Model file for the job. Use its own axes, mm. A direction names the side the tool comes from. Coordinates: 2 decimals unless noted, no trailing zeros. Write each loop counter-clockwise with the first axis right and the second up, starting at its lowest first coordinate (ties: lowest second). Pieces come first, ordered by that corner, then holes.
Q1. Band-saw the part on B-B, the plane x = -2. Write the cut outline in (y, z).
Q2. Band-saw the part on D-D, the plane x = 9.5. Write the cut outline in (y, z).
Q3. Pin check, flat tips, straight feed: P1, Ø6, axis at y = 16, z = -14, coming from the +X side; P2, Ø1.5, axis at x = 13.5, z = 7, coming from the +Y side; P3, Ø4, axis at y = 13.5, z = -22.5, coming from the -X side. Stop position of each tip, or through.
Q4. Band-saw the part on C-C, the plane z = -21. Write the cut outline in (x, y), plus the area to 3 significant figures.
Q5. Pull direction X, two halves, no side cores. Call faces 1 (the cylindrical face through (-29.4, 15.18, 29.43)), 2 (the flat face through (0, 1.5, 0)), 3 (the cylindrical face through (29.43, 15.18, 29.4)), 4 (the flat face through (-31, 2, -1)): released by +X, released by -X, zero draft, split by the parting line, or undercut.
Q6. Drill centre lines: probe 1 along Z at (x, y) = (-19.5, 11); probe 2 along Y at (x, z) = (23, 11). Where is each one in solid material? Low to high.
Q7. Which spindle directions (+Z, -Z, +X, -X, +Y, -Y) get a long thin tool onto all of the face, cutting with end or side? Do faces 5 (the flat face through (0, 15, 30)), 6 (the flat face through (0, 15, -28.5)), 7 (the flat face through (31, 2, -1)). Say none if no direction does.
from build123d import *

# Parameters (mm, degrees)
SKETCH_1_W            = 60
SKETCH_1_H            = 60
EXTRUDE_1_DEPTH       = 28
SKETCH_2_W            = 57
SKETCH_2_H            = 57
CUT_EXTRUDE_1_DEPTH   = 26.5
EXTRUDE_3_DEPTH       = 26
MIRROR_5_COPY_1_DEPTH = 26
SKETCH_4_W            = 8
SKETCH_4_H            = 2
CUT_EXTRUDE_2_DEPTH   = 2
FILLET_1_R            = 2


with BuildPart() as part:
    # 草图1 → 凸台-拉伸1 (new body)
    with BuildSketch(Plane(origin=(0, 0, 0), x_dir=(1, 0, 0), z_dir=(0, 1, 0))):
        Rectangle(SKETCH_1_W, SKETCH_1_H)
    extrude(amount=EXTRUDE_1_DEPTH)

    # 草图2 → 切除-拉伸1 (cut)
    with BuildSketch(Plane(origin=(0, 28, 0), x_dir=(1, 0, 0), z_dir=(0, 1, 0))):
        Rectangle(SKETCH_2_W, SKETCH_2_H)
    extrude(amount=-CUT_EXTRUDE_1_DEPTH, mode=Mode.SUBTRACT)

    # 草图3 → 凸台-拉伸3 (add)
    with BuildSketch(Plane(origin=(0, 28, 0), x_dir=(1, 0, 0), z_dir=(0, 1, 0))):
        with BuildLine():
            Line((-30, 0), (-30, -1.5))
            Line((-30, -1.5), (-30.677124344, -1.5))
            ThreePointArc((-30.677124344, -1.5), (-31.088161527, -1.780042303), (-31.555590279, -1.95))
            Line((-31.555590279, -1.95), (-32.5, -1.95))
            Line((-32.5, -1.95), (-32.5, -1.443375673))
            Line((-32.5, -1.443375673), (-30, 0))
        make_face()
    extrude_3 = extrude(amount=-EXTRUDE_3_DEPTH)

    # 镜向4: 凸台-拉伸3 across plane
    add(extrude_3.mirror(Plane.XY))

    # 镜向5: 凸台-拉伸3 across plane
    add(extrude_3.mirror(Plane(origin=(0, 0, 0), x_dir=(0, 0, 1), z_dir=(1, 0, 0))))

    # 镜向5 copy 1 sketch → 镜向5 copy 1 (add)
    with BuildSketch(Plane(origin=(0, 28, 0), x_dir=(-1, 0, 0), z_dir=(0, 1, 0))):
        with BuildLine():
            Line((-30, 0), (-30, -1.5))
            Line((-30, -1.5), (-30.677124344, -1.5))
            ThreePointArc((-30.677124344, -1.5), (-31.088161527, -1.780042303), (-31.555590279, -1.95))
            Line((-31.555590279, -1.95), (-32.5, -1.95))
            Line((-32.5, -1.95), (-32.5, -1.443375673))
            Line((-32.5, -1.443375673), (-30, 0))
        make_face()
    extrude(amount=-MIRROR_5_COPY_1_DEPTH)

    # 草图4 → 切除-拉伸2 (cut)
    with BuildSketch(Plane(origin=(0, 28, 0), x_dir=(1, 0, 0), z_dir=(0, 1, 0))):
        with Locations((0, -30)):
            Rectangle(SKETCH_4_W, SKETCH_4_H)
    extrude(amount=-CUT_EXTRUDE_2_DEPTH, mode=Mode.SUBTRACT)

    # 圆角1
    fillet_1_edges = [part.edges().sort_by_distance(p)[0] for p in [
        (-30, 0, 0),
        (0, 0, 30),
        (30, 0, 0),
        (0, 0, -30),
        (30, 14, 30),
        (-30, 14, 30),
        (30, 14, -30),
        (-30, 14, -30),
    ]]
    fillet(fillet_1_edges, radius=FILLET_1_R - 0.0001)  # a hair under: the kernel refuses the full size


solid = part.part
Answer sheet:
1. outline: (0, -28) arc R2 ccw to (2, -30) - (28, -30) - (28, -28.5) - (1.5, -28.5) - (1.5, 28.5) - (28, 28.5) - (28, 29) - (26, 29) - (26, 30) - (2, 30) arc R2 ccw to (0, 28) - close
2. outline: (0, -28) arc R2 ccw to (2, -30) - (28, -30) - (28, -28.5) - (1.5, -28.5) - (1.5, 28.5) - (28, 28.5) - (28, 30) - (2, 30) arc R2 ccw to (0, 28) - close
3. P1: stops at x = 30
3. P2: stops at y = 1.5
3. P3: stops at x = -30
4. outline: (-30, 2) arc R2 ccw to (-28, 0) - (28, 0) arc R2 ccw to (30, 2) - (30, 28) - (28.5, 28) - (28.5, 1.5) - (-28.5, 1.5) - (-28.5, 28) - (-30, 28) - close
4. area: 168 mm2
5. face 1: released by -X
5. face 2: undercut
5. face 3: released by +X
5. face 4: zero draft
6. probe 1: z = -30 to -28.5, 28.5 to 30
6. probe 2: y = 0 to 1.5
7. face 5: +Z, +X, -X, +Y, -Y
7. face 6: +Y
7. face 7: +Z, -Z, +X, -Y
